Autodesk Inventor part; units mm, degrees
ref_plane "IDS_WORKPLANE{1}" through (-5.4864, 0, 0) normal (1, 0, 0) x (0, 0, -1)
ref_plane "Work Plane2" through (41.275, 0, 0) normal (0, 0, -1) x (1, 0, 0)
ref_plane "YZ Plane" through (0, 0, 0) normal (1, 0, 0) x (0, 1, 0)
sketch "Sketch1" plane through (0, 0, 0) normal (0, 0, 1) x (1, 0, 0)
  line L0 (-5.4864, 0) -> (19.05, 0)
  line L1 (19.05, 0) -> (19.05, 3.175)
  line L2 (19.05, 3.175) -> (3.175, 3.175)
  line L3 (3.175, 3.175) -> (2.413, 3.175)
  line L4 (2.413, 3.175) -> (0, 3.175)
  line L5 (0, 3.175) -> (0, 4.7625)
  line L6 (-10.7699, 0) -> (24.02, 0)
  line L7 (0, -0.9693) -> (0, 5.8158)
  line L8 (0, 4.7625) -> (-4.2103, 4.7625)
  arc A0 (-4.2103, 4.7625) -> (-5.4864, 0) centre (4.0386, 0) ccw
  line L9 (3.175, 3.175) -> (0, 3.175) construction
  dimension "d0" = 19.05
  dimension "d1" = 15.875
  dimension "d2" = 0.762
  dimension "d3" = 5.4864
  dimension "d4" = 6.35
  dimension "d5" = 6.35
  dimension "d9" = 9.525
  dimension "d10" = 0
  dimension "d13" = 9.525
revolve "Body" add sketch "Sketch1" angle 360 about axis through (-5.4864, 0, 0) along (1, 0, 0)
ref_plane "IDS_WORKPLANE{1}" through (-5.4864, 0, 0) normal (1, 0, 0) x (0, 0, -1)
sketch "Sketch2" plane through (-5.4864, 0, 0) normal (1, 0, 0) x (0, 0, -1)
  circle A0 centre (0, 0) radius 4.7625
  line L0 (0, -6.6675) -> (0, 6.6675)
  line L1 (6.6675, 0) -> (-6.6675, 0)
  line L2 (-4.7625, 0.9525) -> (4.7625, 0.9525)
  line L3 (4.7625, 0.9525) -> (4.7625, -0.9525)
  line L4 (4.7625, -0.9525) -> (-4.7625, -0.9525)
  line L5 (-4.7625, -0.9525) -> (-4.7625, 0.9525)
  line L6 (-4.7625, 0) -> (4.7625, 0) construction
  line L7 (0, 0.9525) -> (0, -0.9525) construction
  dimension "d15" = 1.905
extrude "Slot" cut sketch "Sketch2" along normal blind 2.4638 contours L1 L0 L2 A0 | L3 L4 A0 | A0 L4 L0 L1 | A0 L2 L3 | L1 A0 L2 L0 | L0 L4 A0 L1 | L5 L2 A0 | A0 L4 L5
thread "Thread"
sketch "Sketch3" plane through (0, 0, 0) normal (0, 0, 1) x (1, 0, 0)
  line L0 (19.05, 0) -> (19.05, 3.175)
  line L1 (19.05, 3.175) -> (3.175, 3.175)
  line L2 (-5.4864, 0) -> (19.05, 0)
  arc A0 (19.05, 0) -> (18.1993, 3.175) centre (12.7, 0) ccw
  line L3 (19.05, -3.175) -> (19.05, 3.175)
  line L4 (18.1993, 3.175) -> (18.1993, 0)
  line L5 (18.1993, 0) -> (19.05, 0)
  dimension "d40" = 6.35
revolve "Fillet1" cut sketch "Sketch3" angle 360 about axis through (-5.4864, 0, 0) along (1, 0, 0) contours A0 L1 L0
chamfer "Chamfer" distance 0.635 angle 45 1 edges at (18.1993, -3.175, 0)
ref_plane "Work Plane2" through (41.275, 0, 0) normal (0, 0, -1) x (1, 0, 0)
fillet "Fillet4" radius 0.7874 1 edges at (0, -3.175, 0)
equation "\"d0\" = NLG"
equation "\"d1\" = GEL"
equation "\"d2\" = GAL"
equation "\"d3\" = KOH"
equation "\"d4\" = GD"
equation "\"d5\" = BDM"
equation "\"d9\" = KOD"
equation "\"d13\" = KR"
equation "\"d15\" = SBR"
equation "\"d16\" = STI"
equation "\"d40\" = GD"
equation "\"d46\" = R"
equation "\"d11\" = GEL"
equation "\"d43\" = 0.5 * RR"
equation "\"GD\" = NND"
equation "\"NLG\" = 19.05"
equation "\"GEL\" = 15.875"
equation "\"KOD\" = 9.525"
equation "\"KOH\" = 5.4864"
equation "\"GAL\" = 0.762"
equation "\"BDM\" = NND"
equation "\"SBR\" = 1.905"
equation "\"STI\" = 2.4638"
equation "\"KEWI\" = 0"
equation "\"KR\" = KOD"
equation "\"d14\" = -KOH"
equation "\"R\" = 0.7874"
equation "\"THREADDIA\" = 6.35"
equation "\"TOA\" = 30deg"
equation "\"KOH1\" = 4.3688"
equation "\"NND\" = 6.35"
equation "\"GD1\" = 4.8387"
equation "\"THREADDESC\" = 1.2345"
properties part number "ANSI B18.6.2 - 1/4-20 UNC - 0.75, SFHCSI" material "Steel, Mild"
Read the model definition and answer for the solid it produces. Units are mm, in the model's axes. A direction names the side the tool comes from. Round coordinates to 2 decimals unless told otherwise and drop trailing zeros. Write each loop counter-clockwise with the first axis right and the second up, starting at its lowest first coordinate (ties: lowest second). Pieces come first, ordered by that corner, then holes. Notation, with made-up numbers: (45, 52) - (50, 52) arc R29 cw to (50, 76) - close; hole circle Ø7 at (50.5, 32.5). An arc over 180 degrees is marked (long way). Use a Markdown table: item, result.
(1) Which of the six approach directions +Z, -Z, +X, -X, +Y, -Y give full straight-line access (tool end or side, diameter ignored) to faces 1 (the flat face through (-4, -0.952, 0)), 2 (the cylindrical face through (-2.13, -1.03, 4.65))?
Reported:
| item | result |
|---|---|
| face 1 | +Z, -Z, -X |
| face 2 | +X, -X |
(2) The mould has two halves that part along Y. Classify faces 3 (the flat face through (-4, 0.952, 0)), 4 (the flat face through (0, -2, 4)), 5 (the cylindrical face through (9.06, -0.69, 3.1)): released by +Y, released by -Y, zero draft, split by the parting line, or undercut.
Reported:
| item | result |
|---|---|
| face 3 | undercut |
| face 4 | zero draft |
| face 5 | split by the parting line |
(3) The part is cut by section B-B (x = 16). Write down the section's boundary in (y, z) (3 decimals).
Reported:
| item | result |
|---|---|
| outline | circle Ø6.35 at (0, 0) |
(4) Each of these flat-tipped pins is pushed along its axis until it touches: pin 1 Ø3 at (y, z) = (-1.5, -2) entering from +X; pin 2 Ø2 at (x, y) = (0.5, 1) entering from -Z; pin 3 Ø1.2 at (x, z) = (-5, 2) entering from -Y. Where does it stop, or does it pass through?
Reported:
| item | result |
|---|---|
| pin 1 | x = 18.97 |
| pin 2 | z = -4.76 |
| pin 3 | y = -3.97 |
(5) The part is cut by section A-A (x = -0.25). Write down the section's boundary in (y, z) (1 decimal).
Reported:
| item | result |
|---|---|
| outline | circle Ø9.5 at (0, 0) |
(6) Straight lines are drawn through the part: line 1 along X through (y, z) = (1.25, -0.75); line 2 along X through (y, z) = (4.25, -0.5); line 3 along Y through (x, z) = (1.75, -1.5). For each, find the intervals that lie inside material, in ascending order. Write a range as [from, to].
Reported:
| item | result |
|---|---|
| line 1 | [-5.37, 18.88] |
| line 2 | [-4.47, 0] |
| line 3 | [-2.8, 2.8] |
